Here's how the part is built. I have some questions about the finished solid (model axes, mm). Face numbers are marked on the shaded views. A direction names the side the tool comes from. Give positions to 0.01 mm unless a question says otherwise; leave off trailing zeros. Write each loop counter-clockwise with the first axis right and the second up, starting at its lowest first coordinate (ties: lowest second). Pieces come first, ordered by that corner, then holes. Notation, with made-up numbers: (8.5, 14.25) - (56.5, 14.25) arc R14 ccw to (56.5, 32.25) - close; hole circle Ø3 at (31.25, -34.5). An arc over 180 degrees is marked (long way). Use a Markdown table: item, result.
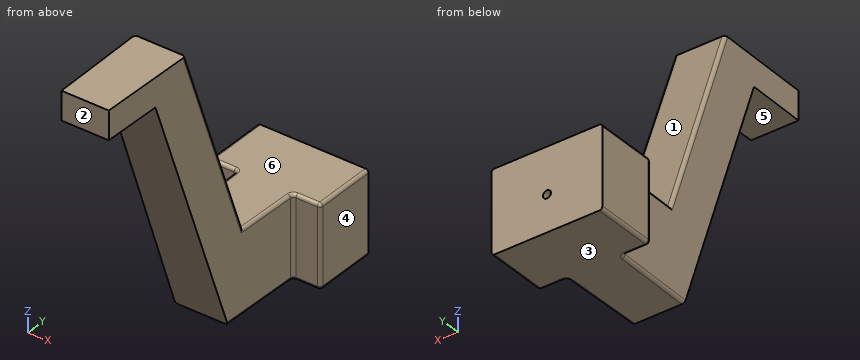
```python
from build123d import *

# Parameters (mm, degrees)
BOSS_EXTRUDE1_DEPTH      = 1.5
SKETCH5_W                = 2.592520813
SKETCH5_H                = 2
BOSS_EXTRUDE2_DEPTH      = 1
BOSS_EXTRUDE2_DEPTH_BACK = 2.5
DRAFT1_ANGLE             = -1
FILLET1_R                = 0.1
SKETCH6_R                = 0.125
CUT_EXTRUDE1_DEPTH       = 2.5


with BuildPart() as part:
    # Sketch1 → Boss-Extrude1 (new body)
    with BuildSketch(Plane(origin=(0, 0, 0), x_dir=(0, 0, -1), z_dir=(1, 0, 0))):
        Polygon((-5.56205373, 1.669569419), (-5.56205373, -0.230430581), (-6.46205373, -0.230430581), (-6.46205373, 2.899223958), (-0.03891584, 5.23705496), (-0.03891584, 9.269569419), (2.553604973, 9.269569419), (2.553604973, 4.623427618), align=None)
    extrude(amount=BOSS_EXTRUDE1_DEPTH)

    # Sketch5 → Boss-Extrude2 (add, two sides)
    with BuildSketch(Plane.ZY) as boss_extrude2_sk:
        with Locations((-1.257344567, 8.269569419)):
            Rectangle(SKETCH5_W, SKETCH5_H)
    extrude(amount=BOSS_EXTRUDE2_DEPTH)
    extrude(boss_extrude2_sk.sketch, amount=-BOSS_EXTRUDE2_DEPTH_BACK)

    # Draft1
    draft1_faces = [part.faces().sort_by_distance(p)[0] for p in [
        (1.5, 4.069973974, 1.641347483),
        (0, 4.069973974, 1.641347483),
    ]]
    draft(draft1_faces, Plane.ZX, DRAFT1_ANGLE)

    # Fillet1
    fillet1_edges = [part.edges().sort_by_distance(p)[0] for p in [
        (-0.10915197, 6.253312189, 0.03891584),
        (-0.071009638, 4.068139459, 3.250484785),
        (1.603796518, 5.946498518, -2.553604973),
        (-0.126890806, 7.269569419, -1.257344566),
        (-0.563445403, 7.269569419, -2.553604973),
        (-0.563445403, 7.269569419, 0.03891584),
        (2.063445403, 7.269569419, -2.553604973),
        (2.5, 8.269569419, -2.553604973),
        (2.5, 8.269569419, 0.03891584),
        (2.063445403, 7.269569419, 0.03891584),
        (1.626890806, 7.269569419, -1.257344566),
        (2.5, 7.269569419, -1.257344566),
        (-1, 8.269569419, -2.553604973),
        (-1, 7.269569419, -1.257344566),
        (-1, 8.269569419, 0.03891584),
        (1.571009638, 4.068139459, 3.250484785),
        (1.60915197, 6.253312189, 0.03891584),
        (-0.103796518, 5.946498518, -2.553604973),
    ]]
    fillet(fillet1_edges, radius=FILLET1_R)

    # Sketch6 → Cut-Extrude1 (cut)
    with BuildSketch(Plane(origin=(0, 9.269569419, 0), x_dir=(1, 0, 0), z_dir=(0, 1, 0))):
        with Locations((0.75, 1.403604973)):
            Circle(SKETCH6_R)
    extrude(amount=-CUT_EXTRUDE1_DEPTH, mode=Mode.SUBTRACT)


solid = part.part
```
Item 1: I need wall thicknesses on line 1 along Z through (x, y) = (0.75, 8.65); line 2 along Y through (x, z) = (-0.4, -0.25); line 3 along Z through (x, y) = (0.85, 0.5). Which ranges of each line are inside material? Lowest first, please. Write a range as [from, to].
Values:
| item | result |
|---|---|
| line 1 | z = [-2.55, -1.53], [-1.28, 0.04] |
| line 2 | y = [7.27, 9.27] |
| line 3 | z = [5.56, 6.46] |
Item 2: If we section it at B-B, the plane x = 0.75: Write out the boundary of the cut face in (y, z).
Values:
| item | result |
|---|---|
| outline | (-0.23, 5.56) - (1.67, 5.56) - (4.62, -2.55) - (9.27, -2.55) - (9.27, -1.53) - (6.77, -1.53) - (6.77, -1.28) - (9.27, -1.28) - (9.27, 0.04) - (5.24, 0.04) - (2.9, 6.46) - (-0.23, 6.46) - close |
Item 3: Thinking about a two-plate mould opening in Y: for the marked faces 1, 2 and 3, which applies, +Y half, -Y half, draft (parallel to the pull), parting line (faces both ways), or undercut?
Values:
| item | result |
|---|---|
| face 1 | +Y half |
| face 2 | -Y half |
| face 3 | draft |
Item 4: If we section it at C-C, the plane y = 2.5: Write out the boundary of the cut face in (x, z).
Values:
| item | result |
|---|---|
| outline | (-0.04, 3.28) - (1.54, 3.28) - (1.54, 6.46) - (-0.04, 6.46) - close |
Item 5: Will these pins go through, and if not, where does the flat tip stop? pin 1 Ø1.2 at (x, y) = (1, 0.5) entering from -Z; pin 2 Ø0.5 at (x, z) = (-0.5, -1.5) entering from -Y; pin 3 Ø1 at (x, z) = (1, 3.5) entering from -Y.
Values:
| item | result |
|---|---|
| pin 1 | stops at z = 5.56 |
| pin 2 | stops at y = 7.27 |
| pin 3 | stops at y = 2.24 |
Item 6: If we section it at A-A, the plane y = 7.5: Write out the boundary of the cut face in (x, z) (3 decimals).
Values:
| item | result |
|---|---|
| outline | (-1, -2.454) arc R0.1 ccw to (-0.9, -2.554) - (2.4, -2.554) arc R0.1 ccw to (2.5, -2.454) - (2.5, -0.061) arc R0.1 ccw to (2.4, 0.039) - (-0.9, 0.039) arc R0.1 ccw to (-1, -0.061) - close; hole circle Ø0.25 at (0.75, -1.404) |
Item 7: For the marked faces 4, 5 and 6, which set-ups out of +Z, -Z, +X, -X, +Y, -Y let a thin tool reach every point of the face, with its end or its side?
Values:
| item | result |
|---|---|
| face 4 | +Z, -Z, +X, +Y, -Y |
| face 5 | -Z, +X, -X, -Y |
| face 6 | +Z, +X, -X, +Y |
Item 8: If we section it at D-D, the plane x = -0.4: Write out the boundary of the cut face in (y, z).
Values:
| item | result |
|---|---|
| outline | (7.27, -2.45) arc R0.1 ccw to (7.37, -2.55) - (9.27, -2.55) - (9.27, 0.04) - (7.37, 0.04) arc R0.1 ccw to (7.27, -0.06) - close |
